Check sheet for the drawn part. Datum: minimum x, y, z corner. Units: mm. A direction names the side the tool comes from. Coordinates: 2 decimals unless noted, no trailing zeros. Write each loop counter-clockwise with the first axis right and the second up, starting at its lowest first coordinate (ties: lowest second). Pieces come first, ordered by that corner, then holes. Notation, with made-up numbers: M 78,-36.75 L 96,-36.75 A17 ccw 96,-21.75 Z; hole C 41,-7.75 d6. An arc over 180 degrees is marked long. Answer in a Markdown table with one row per item.
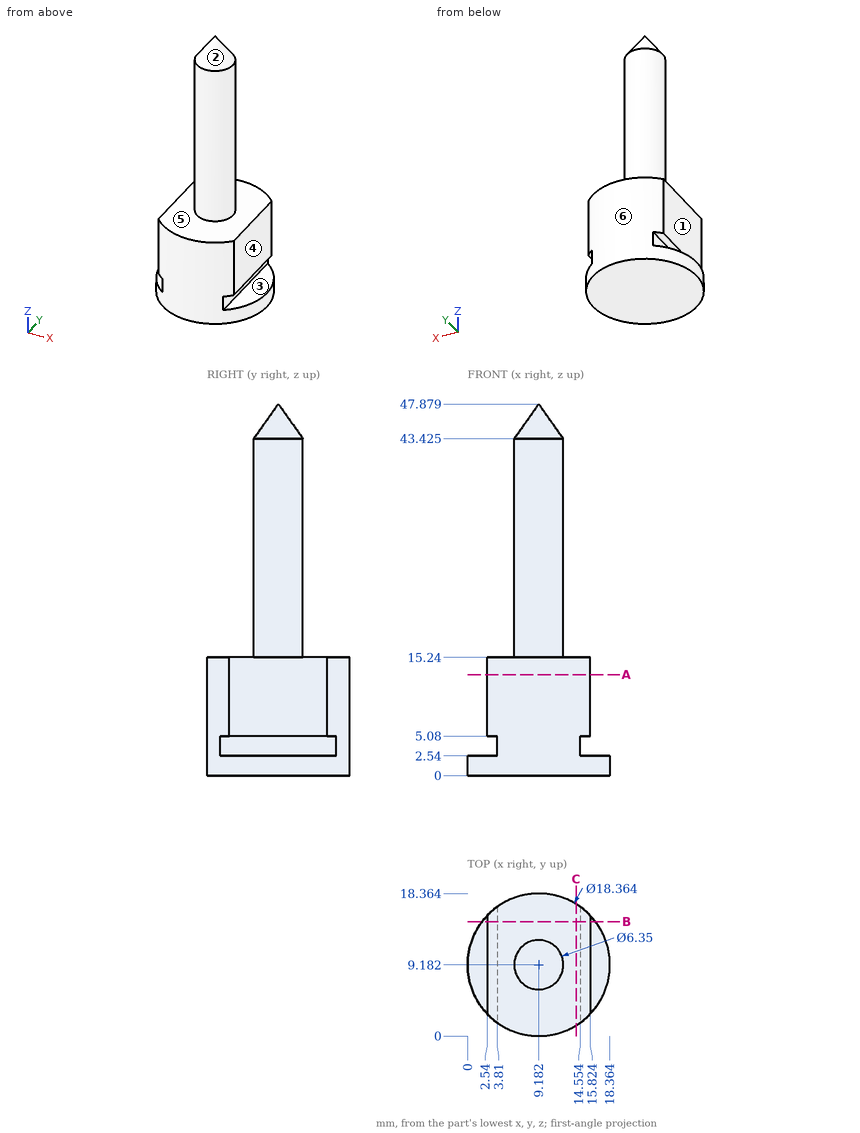
1) Release check for a two-part mould opening along Z. For the marked faces 1, 2 and 3 record: +Z half, -Z half, draft (parallel to the pull), parting line (faces both ways), or undercut.
Response values:
| item | result |
|---|---|
| face 1 | draft |
| face 2 | +Z half |
| face 3 | undercut |
2) Tool access check on the marked faces 4, 5 and 6. Record the directions out of +Z, -Z, +X, -X, +Y, -Y that give a thin tool (end or side, any length) a straight path to the whole face; none if there is none.
Response values:
| item | result |
|---|---|
| face 4 | +Z, +X, +Y, -Y |
| face 5 | +Z |
| face 6 | +Z, -Z |
3) Thickness scan on L1, parallel to Z at x = 15.5, y = 11; L2, parallel to Y at x = 9, z = 32; L3, parallel to Z at x = 16, y = 11.25. Record the ranges inside material, lowest first. Write a range as [from, to].
Response values:
| item | result |
|---|---|
| L1 | z = [0, 2.54], [5.08, 15.24] |
| L2 | y = [6.01, 12.35] |
| L3 | z = [0, 2.54] |
4) Sectioned sample at C-C (x = 14). Record the cut outline in (y, z) (1 decimal), then the cut area to 3 significant figures.
Response values:
| item | result |
|---|---|
| outline | M 1.4,0 L 17,0 L 17,15.2 L 1.4,15.2 Z |
| area | 238 mm² |
5) Sectioned sample at B-B (y = 14.75). Record the cut outline in (x, z) (1 decimal), then the cut area to 3 significant figures.
Response values:
| item | result |
|---|---|
| outline | M 1.9,0 L 16.5,0 L 16.5,2.5 L 14.6,2.5 L 14.6,5.1 L 15.8,5.1 L 15.8,15.2 L 2.5,15.2 L 2.5,5.1 L 3.8,5.1 L 3.8,2.5 L 1.9,2.5 Z |
| area | 199 mm² |
6) Sectioned sample at A-A (z = 13). Record the cut outline in (x, y) (1 decimal), then the cut area to 3 significant figures.
Response values:
| item | result |
|---|---|
| outline | M 2.5,2.8 A9.2 ccw 15.8,2.8 L 15.8,15.5 A9.2 ccw 2.5,15.5 Z |
| area | 221 mm² |
7) Depth check by flat-ended pin: pin 1 (3 mm diameter, centred on x = 4, y = 16, fed in from +Z); pin 2 (5 mm diameter, centred on x = 2, z = 18, fed in from +Y); pin 3 (4 mm diameter, centred on y = 6.5, z = 39.5, fed in from +X); pin 4 (5 mm diameter, centred on x = 4, z = 33, fed in from +Y). Enter the tip coordinate at first touch or a pass-through.
Response values:
| item | result |
|---|---|
| pin 1 | stops at z = 15.24 |
| pin 2 | passes through |
| pin 3 | stops at x = 12.28 |
| pin 4 | stops at y = 10.88 |
